Autodesk Inventor part; units mm, degrees
ref_plane "YZ Plane" through (0, 0, 0) normal (1, 0, 0) x (0, 1, 0)
ref_plane "XZ Plane" through (0, 0, 0) normal (0, 1, 0) x (-1, 0, 0)
ref_plane "XY Plane" through (0, 0, 0) normal (0, 0, 1) x (1, 0, 0)
sketch "Sketch4" plane through (0, 0, 0) normal (0, 0, 1) x (1, 0, 0)
  line L0 (107.5, 20) -> (-107.5, 20)
  line L1 (-107.5, -20) -> (107.5, -20)
  line L2 (107.5, -20) -> (-107.5, 20) construction
  line L3 (107.5, 20) -> (-107.5, -20) construction
  circle A0 centre (-107.5, 0) radius 5.5
  arc A1 (-107.5, 20) -> (-107.5, -20) centre (-107.5, 0) ccw
  circle A2 centre (107.5, 0) radius 5.5
  arc A3 (107.5, -20) -> (107.5, 20) centre (107.5, 0) ccw
  point P0 (0, 0)
  dimension "d20" = 40
  dimension "d21" = 215
  dimension "d22" = 11
  dimension "d23" = 11
extrude "Extrusion3" add sketch "Sketch4" along normal blind 10
properties part number "Eslabon"
Geometry check sheet. Reference: the model listing, model coordinates, mm. Coordinates: 2 decimals unless noted, no trailing zeros. Order: outer loops, then holes, each group sorted by start corner. A loop starts at its lowest first (then second) coordinate and runs counter-clockwise, first axis right, second up. Notation, with made-up numbers: M 80.25,-40 L 88.25,-40 A25 cw 88.25,-17 Z; hole C 21,42 d8. An arc over 180 degrees is marked long. Answer as a JSON object with one key per item and string values.
Q1. Scan lines: line 1 (Y direction, x = -107.5, z = 7); line 2 (X direction, y = -1.5, z = 1); line 3 (X direction, y = -4.5, z = 6.5). Record each from-to range of solid material in increasing order.
Results are:
{"line 1": "y = -20 to -5.5, 5.5 to 20", "line 2": "x = -127.44 to -112.79, -102.21 to 102.21, 112.79 to 127.44", "line 3": "x = -126.99 to -110.66, -104.34 to 104.34, 110.66 to 126.99"}
Q2. Release check for a two-part mould opening along Y. For faces 1 (the cylindrical face through (-127.495, -0.44, 4.93)), 2 (the flat face through (-2, -20, 5)), 3 (the cylindrical face through (102, 0, 5)) record: released by +Y, released by -Y, zero draft, split by the parting line, or undercut.
Results are:
{"face 1": "split by the parting line", "face 2": "released by -Y", "face 3": "undercut"}
Q3. Cross-section at C-C on y = 12. Record the cut outline in (x, z).
Results are:
{"outline": "M -123.5,0 L 123.5,0 L 123.5,10 L -123.5,10 Z"}
Q4. Depth check by flat-ended pin: pin 1 Ø9 at (x, y) = (-107.5, 0) entering from -Z; pin 2 Ø5 at (y, z) = (-11.5, 6.5) entering from +X. Enter the tip coordinate at first touch or a pass-through.
Results are:
{"pin 1": "passes through", "pin 2": "stops at x = 125.36"}
Q5. Cross-section at A-A on y = 0. Record the cut outline in (x, z), and give its area (3 significant figures).
Results are:
{"outline": "M -127.5,0 L -113,0 L -113,10 L -127.5,10 Z; M -102,0 L 102,0 L 102,10 L -102,10 Z; M 113,0 L 127.5,0 L 127.5,10 L 113,10 Z", "area": "2,330 mm²"}
Q6. Cross-section at B-B on z = 3.75. Record the cut outline in (x, y), and give its area (3 significant figures).
Results are:
{"outline": "M -107.5,-20 L 107.5,-20 A20 ccw 107.5,20 L -107.5,20 A20 ccw Z; hole C -107.5,0 d11; hole C 107.5,0 d11", "area": "9,670 mm²"}
